Geometry: see drawing. Coordinates: mm, zero at the bounding-box minimum. A direction names the side the tool comes from. Round coordinates to 2 decimals unless told otherwise and drop trailing zeros. Loops run counter-clockwise (first coordinate to the right, second up) from the corner with the lowest first, then second, coordinate; pieces in that order, holes last. Notation, with made-up numbers: M -7,-10 L 39,-10 A29 cw 39,27 Z; hole C -30,-37.5 d4. An arc over 180 degrees is marked long. Answer as a JSON object with one key per item and string values.
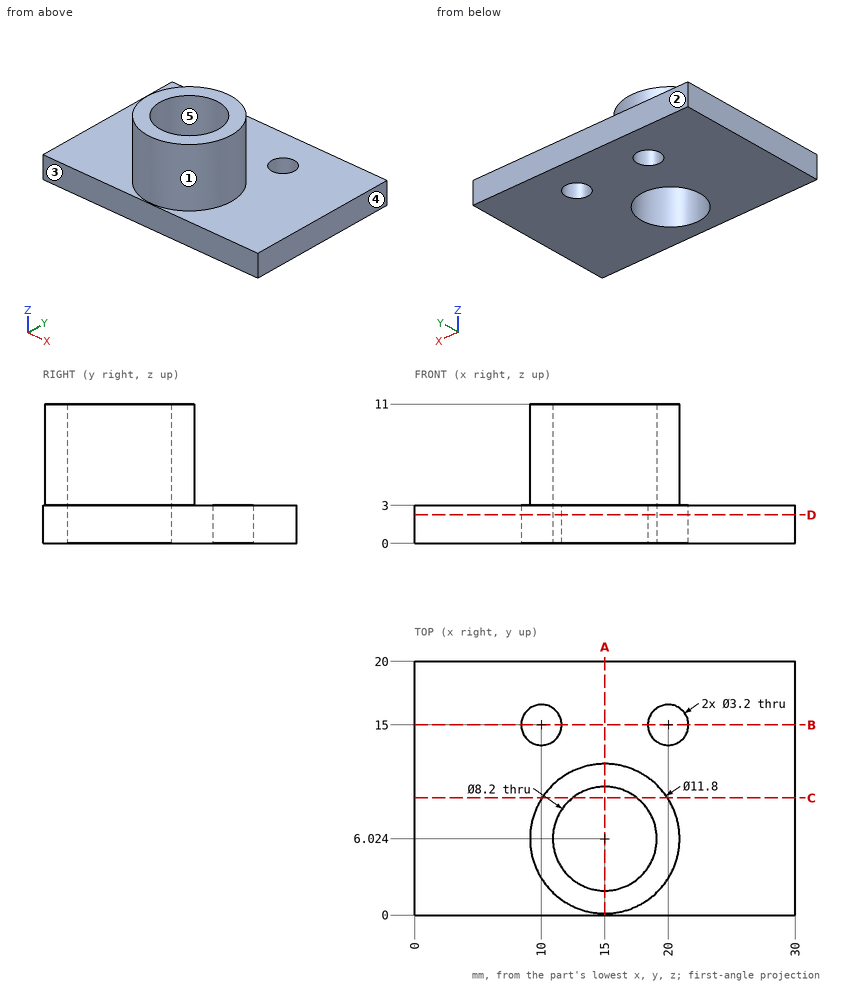
1) Section query A-A (x = 15). Return the cut outline in (y, z), and give its area (3 significant figures).
Results:
{"outline": "M 0,0 L 1.92,0 L 1.92,11 L 0.12,11 L 0.12,3 L 0,3 Z; M 10.12,0 L 20,0 L 20,3 L 11.92,3 L 11.92,11 L 10.12,11 Z", "area": "64.2 mm2"}
2) Reachability of the marked faces 1 and 2 from +Z, -Z, +X, -X, +Y, -Y: full face, straight path, thin tool, end or side. Return the list, or none.
Results:
{"face 1": "+Z", "face 2": "+Z, -Z, +X, -X, +Y"}
3) Pull-direction query (X, two-part tool) for the marked faces 3, 4 and 5; classes: +X half, -X half, draft (parallel to the pull), parting line (faces both ways), or undercut.
Results:
{"face 3": "draft", "face 4": "+X half", "face 5": "undercut"}
4) Pin query (flat end, axial travel): P1, Ø3, axis at y = 5.5, z = 2.5, coming from the -X side; P2, Ø1.9, axis at x = 10, y = 15, coming from the +Z side; P3, Ø2, axis at y = 10, z = 7.5, coming from the +X side (1 decimal). Return the tip coordinate at first contact, or that it passes through.
Results:
{"P1": "x = 0", "P2": "through", "P3": "x = 20.1"}
5) Section query C-C (y = 9.25). Return the cut outline in (x, z).
Results:
{"outline": "M 0,0 L 12.47,0 L 12.47,11 L 10.06,11 L 10.06,3 L 0,3 Z; M 17.53,0 L 30,0 L 30,3 L 19.94,3 L 19.94,11 L 17.53,11 Z"}
6) Ray query, line 1 (Z direction, x = 21.5, y = 7.75); line 2 (X direction, y = 6, z = 2.5); line 3 (Y direction, x = 9.75, z = 2.25). Return the intervals inside material, ascending.
Results:
{"line 1": "0 to 3", "line 2": "0 to 10.9, 19.1 to 30", "line 3": "0 to 13.42, 16.58 to 20"}
7) Section query B-B (y = 15). Return the cut outline in (x, z), and give its area (3 significant figures).
Results:
{"outline": "M 0,0 L 8.4,0 L 8.4,3 L 0,3 Z; M 11.6,0 L 18.4,0 L 18.4,3 L 11.6,3 Z; M 21.6,0 L 30,0 L 30,3 L 21.6,3 Z", "area": "70.8 mm2"}
8) Section query D-D (z = 2.25). Return the cut outline in (x, y), and give its area (3 significant figures).
Results:
{"outline": "M 0,0 L 30,0 L 30,20 L 0,20 Z; hole C 10,15 d3.2; hole C 15,6.02 d8.2; hole C 20,15 d3.2", "area": "531 mm2"}
